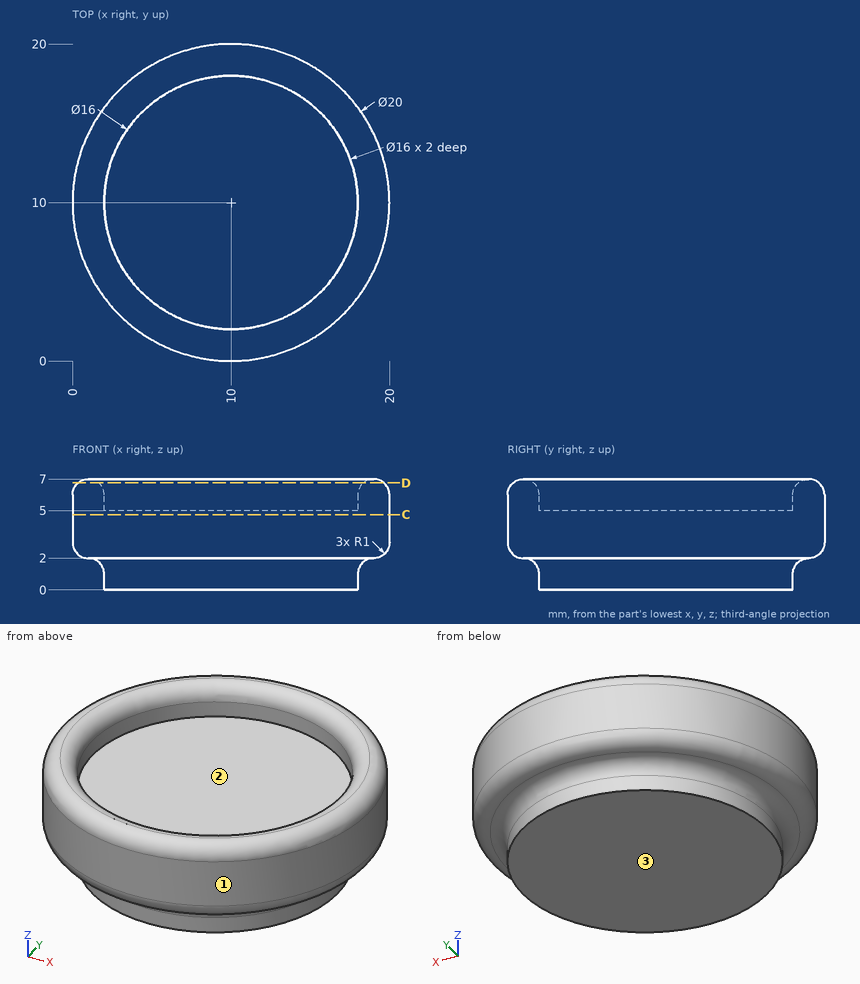
Design review of the part shown in the three views and the two pictorial views. Dimensions are in mm from the part's minimum x, y and z. Round coordinates to 2 decimals unless told otherwise and drop trailing zeros. Loops run counter-clockwise (first coordinate to the right, second up) from the corner with the lowest first, then second, coordinate; pieces in that order, holes last. Notation, with made-up numbers: (47, 78.5) -> (79, 78.5) arc R28 ccw to (79, 105.5) -> close; hole circle Ø5 at (9.5, 37.5). An arc over 180 degrees is marked (long way). Answer as a JSON object with one key per item and string values. Group by question number.
1) For line 1 (Y direction, x = 10, z = 5.55); line 2 (Y direction, x = 4, z = 3.25); line 3 (Z direction, x = 4, y = 7.5), list the stretches that pass through material, from the lowest coordinate up. Write a range as [from, to].
2) We need section D-D on z = 6.75. Write out the cut boundary in (x, y), then the cut area to 3 significant figures.
3) Mouldability with a two-part tool opening along X and no side actions: class the marked faces 1, 2 and 3 as released by +X, released by -X, zero draft, split by the parting line, or undercut.
4) For pin 1 Ø3 at (x, z) = (14, 1) entering from -Y; pin 2 Ø3 at (x, y) = (5, 8.5) entering from +Z; pin 3 Ø6 at (x, y) = (4.5, 8) entering from -Z, all flat-tipped, find the tip position at first contact; note any pin that passes through.
5) We need section C-C on z = 4.75. Write out the cut boundary in (x, y).
Result set:
{
 "1": {"line 1": "[0, 2], [18, 20]", "line 2": "[2, 18]", "line 3": "[0, 5]"},
 "2": {"outline": "circle Ø19.32 at (10, 10); hole circle Ø16.68 at (10, 10)", "area": "74.8 mm²"},
 "3": {"face 1": "split by the parting line", "face 2": "undercut", "face 3": "zero draft"},
 "4": {"pin 1": "y = 0.83", "pin 2": "z = 5", "pin 3": "z = 0"},
 "5": {"outline": "circle Ø20 at (10, 10)"}
}
